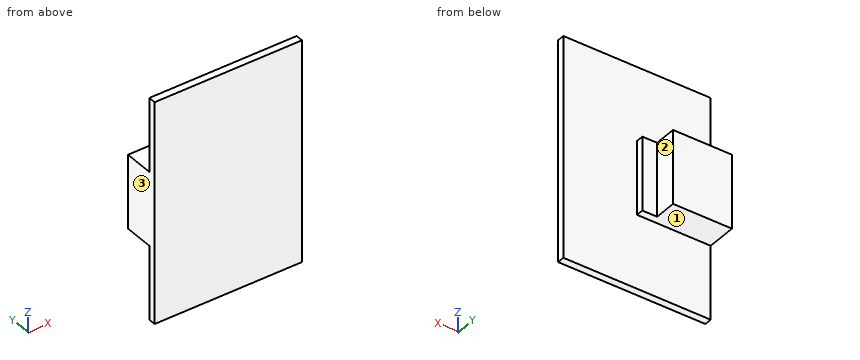
```python
from build123d import *

# Parameters (mm, degrees)
SCHIZZO1_W                   = 8
SCHIZZO1_H                   = 10
ESTRUSIONE_ESTRUSIONE1_DEPTH = 5
SCHIZZO2_W                   = 10
SCHIZZO2_H                   = 2
ESTRUSIONE_ESTRUSIONE2_DEPTH = 2
SCHIZZO3_W                   = 20
SCHIZZO3_H                   = 30
ESTRUSIONE_ESTRUSIONE3_DEPTH = 1


with BuildPart() as part:
    # Schizzo1 → Estrusione-Estrusione1 (new body)
    with BuildSketch(Plane(origin=(0, 0, 0), x_dir=(1, 0, 0), z_dir=(0, 1, 0))):
        Rectangle(SCHIZZO1_W, SCHIZZO1_H)
    extrude(amount=ESTRUSIONE_ESTRUSIONE1_DEPTH)

    # Schizzo2 → Estrusione-Estrusione2 (add)
    with BuildSketch(Plane(origin=(4, 0, 0), x_dir=(0, 0, -1), z_dir=(1, 0, 0))):
        with Locations((0, 1)):
            Rectangle(SCHIZZO2_W, SCHIZZO2_H)
    extrude(amount=ESTRUSIONE_ESTRUSIONE2_DEPTH)

    # Schizzo3 → Estrusione-Estrusione3 (add)
    with BuildSketch(Plane.XZ):
        with Locations((6, 0)):
            Rectangle(SCHIZZO3_W, SCHIZZO3_H)
    extrude(amount=-ESTRUSIONE_ESTRUSIONE3_DEPTH)


solid = part.part
```
Verification items for the finished model (mm, model axes). Face numbers are marked on the shaded views. A direction names the side the tool comes from. Give positions to 0.01 mm unless a question says otherwise; leave off trailing zeros. Order: outer loops, then holes, each group sorted by start corner. A loop starts at its lowest first (then second) coordinate and runs counter-clockwise, first axis right, second up. Notation, with made-up numbers: M 60.25,4 L 89.25,4 A18 cw 89.25,31 Z; hole C -13.5,74.25 d10. An arc over 180 degrees is marked long. Answer in a Markdown table with one row per item. Add a question column.
Item 1: Section check B-B, the plane x = -2.25. Enter the section's corners in (y, z), and give its area (3 significant figures).
Item 2: Section check C-C, the plane y = 1.45. Enter the section's corners in (x, z), and give its area (3 significant figures).
Item 3: Tool access check on the marked faces 1, 2 and 3. Record the directions out of +Z, -Z, +X, -X, +Y, -Y that give a thin tool (end or side, any length) a straight path to the whole face; none if there is none.
Item 4: Section check A-A, the plane z = 3.25. Enter the section's corners in (x, y).
Item 5: Scan lines: probe 1 along Y at (x, z) = (1.75, -12); probe 2 along Z at (x, y) = (2.25, 2.05); probe 3 along X at (y, z) = (1.35, -4.75). Record each from-to range of solid material in increasing order. Write a range as from..to.
Item 6: Section check D-D, the plane x = 10. Enter the section's corners in (y, z).
Item 7: Gauge pin test, flat ends, axial feed: pin 1 (1.5 mm diameter, centred on y = 2.5, z = -6, fed in from +X); pin 2 (2.5 mm diameter, centred on y = 3, z = 1.5, fed in from +X); pin 3 (1 mm diameter, centred on x = 5.5, z = -1, fed in from +Y); pin 4 (2 mm diameter, centred on x = 3.5, y = 3, fed in from +Z). Record the tip position at first contact, or that the pin passes through.
Filled sheet:
| question | item | result |
|---|---|---|
| 1 | outline | M 0,-15 L 1,-15 L 1,-5 L 5,-5 L 5,5 L 1,5 L 1,15 L 0,15 Z |
| 1 | area | 70.0 mm^2 |
| 2 | outline | M -4,-5 L 6,-5 L 6,5 L -4,5 Z |
| 2 | area | 100 mm^2 |
| 3 | face 1 | -Z, +X, -X, +Y |
| 3 | face 2 | +Z, -Z, +X, +Y |
| 3 | face 3 | +Z, -Z, -X, +Y, -Y |
| 4 | outline | M -4,0 L 16,0 L 16,1 L 6,1 L 6,2 L 4,2 L 4,5 L -4,5 Z |
| 5 | probe 1 | y = 0..1 |
| 5 | probe 2 | z = -5..5 |
| 5 | probe 3 | x = -4..6 |
| 6 | outline | M 0,-15 L 1,-15 L 1,15 L 0,15 Z |
| 7 | pin 1 | passes through |
| 7 | pin 2 | stops at x = 6 |
| 7 | pin 3 | stops at y = 2 |
| 7 | pin 4 | stops at z = 5 |
